Autodesk Fusion 360 part; units mm, degrees
sketch "Sketch1" plane through (0, 0, 0) normal (0, 0, 1) x (1, 0, 0)
  line L0 (0, 50) -> (53.404, 50)
  line L1 (54, -38) -> (0, -38)
  line L2 (0, -38) -> (0, 50)
  arc A0 (54, -38) -> (63.0412, -34.3412) centre (54, -25) ccw
  arc A1 (62.6413, 46.1473) -> (53.404, 50) centre (53.404, 37) ccw
  line L3 (63.0412, -34.3412) -> (89.552, -7.4343)
  line L4 (89.4528, 19.3358) -> (62.6413, 46.1473)
  arc A2 (89.552, -7.4343) -> (89.4528, 19.3358) centre (76.0178, 5.9008) ccw
  circle A3 centre (31, -24) radius 5
  circle A4 centre (31, 36) radius 5
  dimension "d2" = 88
  dimension "d6" = 13
  dimension "d7" = 13
  dimension "d10" = 19
  dimension "d13" = 10
  dimension "d15" = 10
extrude "Extrude1" add sketch "Sketch1" along normal blind 10 makes body 1
sketch "Sketch2" plane through (0, 0, 10) normal (0, 0, 1) x (-1, 0, 0)
  circle A0 centre (-31, -36) radius 5
  circle A1 centre (-31, 24) radius 5
  arc A2 (-54, 38) -> (-63.0412, 34.3412) centre (-54, 25) ccw
  line L0 (-63.0412, 34.3412) -> (-89.552, 7.4343)
  arc A3 (-89.552, 7.4343) -> (-89.4528, -19.3358) centre (-76.0178, -5.9008) ccw
  line L1 (-89.4528, -19.3358) -> (-62.6413, -46.1473)
  arc A4 (-62.6413, -46.1473) -> (-53.404, -50) centre (-53.404, -37) ccw
  line L2 (-53.404, -50) -> (0, -50)
  line L3 (0, -50) -> (0, 38)
  line L4 (0, 38) -> (-54, 38)
  line L5 (0, 38) -> (-13, 38)
  line L6 (-13, 38) -> (-13, 16)
  line L7 (0, 13) -> (0, 38)
  line L8 (0, -50) -> (-13, -50)
  line L9 (-13, -50) -> (-13, -28)
  line L10 (0, -25) -> (0, -50)
  line L11 (-13, -25) -> (-16, -25)
  line L12 (-16, -25) -> (-16, -25)
  line L13 (25, -25) -> (25, 13)
  line L14 (-16, 13) -> (-16, 13)
  line L15 (-16, 13) -> (-16, -25)
  arc A5 (-16, 13) -> (-13, 16) centre (-16, 16) ccw
  arc A6 (-13, -28) -> (-16, -25) centre (-16, -28) ccw
  line L16 (25, 13) -> (6, 13)
  line L17 (25, -25) -> (0, -25)
  line L18 (0, -50) -> (0, -31)
  line L19 (6, -25) -> (25, -25)
  line L20 (25, -25) -> (25, 13)
  line L21 (25, 13) -> (0, 13)
  line L22 (0, 19) -> (0, 38)
  arc A7 (0, 19) -> (6, 13) centre (6, 19) ccw
  arc A8 (6, -25) -> (0, -31) centre (6, -31) ccw
  dimension "d18" = 13
  dimension "d19" = 25
  dimension "d20" = 13
  dimension "d21" = 25
  dimension "d23" = 41
  dimension "d24" = 3
  dimension "d25" = 3
  dimension "d26" = 6
  dimension "d27" = 6
extrude "Extrude2" add sketch "Sketch2" against normal blind 10 contours L3 L7 L21 A7 | L3 L13 L16 L17 L19 L20 L21 | L3 L10 L17 A8 bodies 1
extrude "Extrude3" add sketch "Sketch2" along normal blind 30 contours L3 L7 L21 A7 | L3 L13 L16 L17 L19 L20 L21 | L3 L10 L17 A8 bodies 1
extrude "Extrude4" add sketch "Sketch2" along normal blind 30 contours L2 L3 L4 L5 L6 L7 L8 L9 L10 L15 A5 A6 L18 L22 bodies 1
fillet "Fillet1" radius 19 2 edges at (-25, -13, 20) (-25, 25, 20) on bodies 1
sketch "Sketch3" plane through (0, 0, 40) normal (0, 0, 1) x (-1, 0, 0)
  arc A0 (6, -25) -> (25, -6) centre (6, -6) ccw
  arc A1 (25, -6) -> (6, 13) centre (6, -6) ccw
  arc A2 (0, 19) -> (6, 13) centre (6, 19) ccw
  line L0 (0, 19) -> (0, 38)
  line L1 (0, 38) -> (-13, 38)
  line L2 (-13, 38) -> (-13, 16)
  arc A3 (-16, 13) -> (-13, 16) centre (-16, 16) ccw
  line L3 (-16, 13) -> (-16, -25)
  arc A4 (-13, -28) -> (-16, -25) centre (-16, -28) ccw
  line L4 (-13, -28) -> (-13, -50)
  line L5 (-13, -50) -> (0, -50)
  line L6 (0, -50) -> (0, -31)
  arc A5 (6, -25) -> (0, -31) centre (6, -31) ccw
  circle A6 centre (6, -6) radius 9.5
  dimension "d36" = 19
extrude "Extrude5" cut sketch "Sketch3" against normal blind 40 contours A6 bodies 1
sketch "Sketch4" plane through (0, -38, 0) normal (0, -1, 0) x (1, 0, 0)
  line L0 (0, 0) -> (54, 0)
  line L1 (54, 0) -> (54, 10)
  line L2 (54, 10) -> (13, 10)
  line L3 (13, 10) -> (13, 40)
  line L4 (13, 40) -> (0, 40)
  line L5 (0, 40) -> (0, 0)
  line L6 (16.0173, 10) -> (83.0173, 10)
  line L7 (16.0173, 10) -> (16.0173, 40)
  line L8 (83.0173, 10) -> (16.0173, 40)
  dimension "d39" = 67
  dimension "d40" = 30
extrude "Extrude6" add sketch "Sketch4" along normal blind 10 separate body contours L2 L6 L7 L8 makes body 2
move_body "Move1" bodies 2 to x (1, 0, 0) y (0, 1, 0) z (0, 0, 1) at (0, 49, 0)
combine "Combine1" operation add target body 1 tool bodies 2
Source: CAD feature listing. Evaluate the final solid. Frame: model axes, mm. A direction names the side the tool comes from. Round coordinates to 2 decimals unless told otherwise and drop trailing zeros. Order: outer loops, then holes, each group sorted by start corner. A loop starts at its lowest first (then second) coordinate and runs counter-clockwise, first axis right, second up. Notation, with made-up numbers: (-21.75, 0) - (-1.75, 0) arc R11 ccw to (-1.75, 20) - close; hole circle Ø7 at (-27, 20). An arc over 180 degrees is marked (long way). Use a Markdown table: item, result. Add a question column.
1. Set-up query: faces 1 (the flat face through (34, 11, 19)), 2 (the flat face through (0, -28, 20)), 3 (the flat face through (76.111, -21.076, 4.93)), 4 (the flat face through (53, -3, 10)), 5 (the flat face through (13, -27, 25)). Return all of +Z, -Z, +X, -X, +Y, -Y with unobstructed straight access to the full face (end or side cutting, diameter ignored); none if empty.
2. First-contact query: pin 1 (1.5 mm diameter, centred on y = 8, z = 32, fed in from -X); pin 2 (17.5 mm diameter, centred on y = 37.5, z = 23.5, fed in from +X); pin 3 (2 mm diameter, centred on x = 60, z = 7.5, fed in from -Y). Flat tips, straight axial feed; report the tip coordinate or a pass-through.
3. Section query A-A (z = 35.5). Give the number of separate pieces and of enclosed holes in the cut face, then the cut area to 3 significant figures.
4. Section query B-B (x = 31). Return the cut outline in (y, z), then the cut area to 3 significant figures.
5. Line query: probe 1 along Y at (x, z) = (31, 3); probe 2 along Y at (x, z) = (-6, 25); probe 3 along Z at (x, y) = (75.5, -19.5). Output: solid intervals per line, ascending.
6. Mould query, pull axis X, two halves, no side actions, for faces 6 (the cylindrical face through (95.016, 6.179, 4.93)), 7 (the flat face through (15, 50, 6)), 8 (the cylindrical face through (27, -21, 5)). Classes: +X half, -X half, draft (parallel to the pull), parting line (faces both ways), or undercut.
Derived:
| question | item | result |
|---|---|---|
| 1 | face 1 | +Z, +X, +Y |
| 1 | face 2 | +Z, -Z, -X, -Y |
| 1 | face 3 | +Z, -Z, +X, -Y |
| 1 | face 4 | +Z, +X |
| 1 | face 5 | +Z, +X, -Y |
| 2 | pin 1 | x = -24.96 |
| 2 | pin 2 | x = 13 |
| 2 | pin 3 | y = -37 |
| 3 | separate pieces | 2 |
| 3 | enclosed holes | 1 |
| 3 | area | 1,890 mm2 |
| 4 | outline | (-38, 0) - (-29, 0) - (-29, 10) - (-38, 10) - close; (-19, 0) - (31, 0) - (31, 10) - (11, 10) - (11, 33.29) - (1, 33.29) - (1, 10) - (-19, 10) - close; (41, 0) - (50, 0) - (50, 10) - (41, 10) - close |
| 4 | area | 913 mm2 |
| 5 | probe 1 | -38 to -29, -19 to 31, 41 to 50 |
| 5 | probe 2 | -13 to -3.5, 15.5 to 25 |
| 5 | probe 3 | 0 to 10 |
| 6 | face 6 | +X half |
| 6 | face 7 | draft |
| 6 | face 8 | undercut |
